The listing builds one solid part. Answer for the finished solid, in the listing's coordinates (mm). A direction names the side the tool comes from. Round coordinates to 2 decimals unless told otherwise and drop trailing zeros. Write each loop counter-clockwise with the first axis right and the second up, starting at its lowest first coordinate (ties: lowest second). Pieces come first, ordered by that corner, then holes.
Item 1: Find the intervals of material crossed by probe 1 along Z at (x, y) = (-1, 0.55); probe 2 along X at (y, z) = (1.5, 0.6); probe 3 along Y at (x, z) = (9, -0.45), in increasing order.
Item 2: For a pull along Y with two mould halves and no side action, classify faces 3 (the face through (4.83, -1.5, -0.07)), 4 (the face through (-0.375, 0.069, -0.022)), 5 (the face through (10, 0, 0)) as +Y half, -Y half, draft (parallel to the pull), parting line (faces both ways), or undercut.
Item 3: A tool of negligible diameter and unlimited length cuts with its end or side. For faces 1 (the face through (-1.7, -1, 1)), 2 (the face through (0, 2, 0)), from which of +Z, -Z, +X, -X, +Y, -Y can it reach the whole face along a straight path? Write none if from no direction.
Item 4: Each of these flat-tipped pins is pushed along its axis until it touches: pin 1 (3 mm diameter, centred on x = 6, y = 0.5, fed in from +Z); pin 2 (1.5 mm diameter, centred on x = 0, y = -1.5, fed in from +Z); pin 3 (0.9 mm diameter, centred on x = -1.5, z = 0, fed in from -Y). Where does it stop, or does it pass through?
Item 5: Find section A-A on x = 1.25. Give the vertices of the cut face in (y, z), then the cut area to 3 significant figures.
Autodesk Inventor part; units mm, degrees
ref_plane "Work Plane1" through (29, 0, 0) normal (0, -1, 0) x (1, 0, 0)
ref_plane "YZ Plane" through (0, 0, 0) normal (1, 0, 0) x (0, 1, 0)
ref_plane "XZ Plane" through (0, 0, 0) normal (0, 1, 0) x (-1, 0, 0)
sketch "Sketch1" plane through (0, 0, 0) normal (0, 0, 1) x (1, 0, 0)
  line L0 (-0.3333, 0) -> (10, 0)
  line L1 (10, 0) -> (10, 1.5)
  line L2 (10, 1.5) -> (7, 1.5)
  line L3 (7, 1.5) -> (6.6932, 1.5)
  line L4 (6.6932, 1.5) -> (0, 1.5)
  line L5 (0, 1.5) -> (0, 2.75)
  line L6 (0, 2.75) -> (-1.7, 2.75)
  line L7 (-1.7, 2.75) -> (-1.7, 1.1547)
  line L8 (-1.7, 1.1547) -> (-1, 1.1547)
  line L9 (-1, 1.1547) -> (-0.3333, 0)
  line L10 (-4.04, 0) -> (12.34, 0)
  line L11 (0, -0.55) -> (0, 3.3)
  line L12 (7, 1.5) -> (0, 1.5) construction
  dimension "d1" = 3
  dimension "d2" = 0.3068
  dimension "d3" = 1.7
  dimension "d4" = 0.7
  dimension "d5" = 60
  dimension "d6" = 3
  dimension "d7" = 3
  dimension "d8" = 2.3094
  dimension "d9" = 5.5
  dimension "d26" = 10
revolve "Body" add sketch "Sketch1" angle 360 about axis through (-0.3333, 0, 0) along (1, 0, 0)
sketch "Sketch2" plane through (-1.7, 0, 0) normal (-1, 0, 0) x (0, 0, 1)
  circle A0 centre (0, 0) radius 1.1547
  line L0 (0, -3.85) -> (0, 3.85)
  line L1 (-3.85, 0) -> (3.85, 0)
  line L2 (1.1547, 0) -> (0.5774, -1)
  line L3 (0.5774, -1) -> (-0.5774, -1)
  line L4 (-0.5774, -1) -> (-1.1547, 0)
  line L5 (-1.1547, 0) -> (-0.5774, 1)
  line L6 (-0.5774, 1) -> (0.5774, 1)
  line L7 (0.5774, 1) -> (1.1547, 0)
extrude "Slot" add sketch "Sketch2" against normal up to next contours L7 A0 | A0 L2 | L6 L0 A0 | A0 L0 L3 | L0 L6 A0 | A0 L3 L0 | L4 A0 | A0 L5
fillet "Fillet1" radius 1 1 edges at (-1.7, -2.75, 0)
chamfer "Chamfer1" distance 0.3067 distance2 0.3067 1 edges at (10, -1.5, 0) measured on face at (10, -0.3743, 0.5709)
ref_plane "Work Plane1" through (29, 0, 0) normal (0, -1, 0) x (1, 0, 0)
fillet "Fillet2" radius 0.1 1 edges at (0, -1.5, 0)
thread "Thread2"
equation "\"d15\" = -0.5 * SPD + 0.5 * GD"
equation "\"d16\" = GUL"
equation "\"GD\" = NND"
equation "\"NLG\" = 6"
equation "\"GEL\" = 4.5"
equation "\"KOD\" = 5.7"
equation "\"KOH\" = 1.65"
equation "\"INTI\" = 1.04"
equation "\"GAL\" = 0.61345 * PTC"
equation "\"GUL\" = 0.61345 * PTC"
equation "\"BDM\" = NND"
equation "\"SW\" = 2"
equation "\"RR\" = 1.45"
equation "\"SPD\" = NND - 1.2269 * PTC"
equation "\"R\" = 0.3"
equation "\"TOA\" = 30deg"
equation "\"GD1\" = THREADDIA - 1.2269 * PTC"
equation "\"THREADDIA\" = 3"
equation "\"PTC\" = 0.5"
equation "\"NND\" = 3"
equation "\"KOH1\" = 0.2"
equation "\"E0\" = 2.303"
properties part number "M3x10 Bolt" material "Stainless Steel"
Check values:
1. probe 1: z = -2.65 to -0.84, 0.84 to 2.65
1. probe 2: x = -1.7 to 0
1. probe 3: y = -1.43 to 1.43
2. face 3: parting line
2. face 4: undercut
2. face 5: draft
3. face 1: +Z, -Z, -X, +Y, -Y
3. face 2: +X
4. pin 1: stops at z = 1.5
4. pin 2: stops at z = 2.65
4. pin 3: stops at y = -2.69
5. outline: circle Ø3 at (0, 0)
5. area: 7.07 mm2
